Source: CAD feature listing. Evaluate the final solid. Frame: model axes, mm. Give positions to 0.01 mm unless a question says otherwise; leave off trailing zeros. Loops run counter-clockwise (first coordinate to the right, second up) from the corner with the lowest first, then second, coordinate; pieces in that order, holes last. Notation, with made-up numbers: M -31,29.5 L -12,29.5 A11 ccw -12,49.5 Z; hole C 57,73.5 d7. An arc over 180 degrees is marked long. Put each result on its own line as item: value.
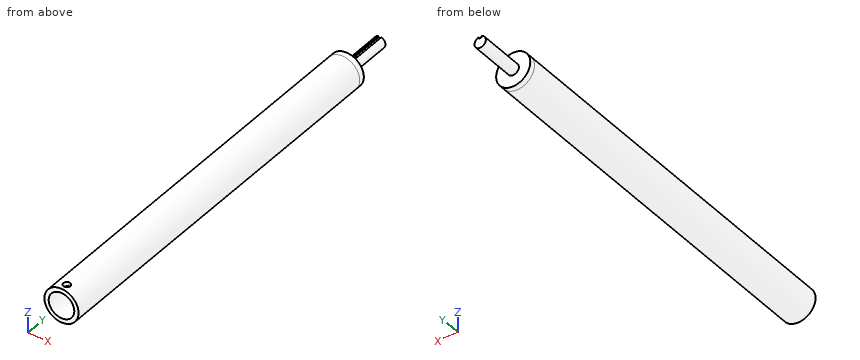
from build123d import *

# Parameters (mm, degrees)
F0_R      = 19.05
F0_R_2    = 14.2875
F1_DEPTH  = 431.8
F2_R      = 19.05
F3_DEPTH  = 6.35
F4_R      = 6.35
F5_DEPTH  = 50.8
F6_W      = 1.6129
F6_H      = 1.778
F7_DEPTH  = 38.1
F10_DEPTH = 9.525


with BuildPart() as f1:
    # F0 (on Front) → F1 (new body)
    with BuildSketch(Plane.XZ):
        Circle(F0_R)
        Circle(F0_R_2, mode=Mode.SUBTRACT)
    extrude(amount=F1_DEPTH)

    # F2 (on face) → F3 (join)
    with BuildSketch(Plane(origin=(0, 0, 0), x_dir=(-1, 0, 0), z_dir=(0, 1, 0))):
        Circle(F2_R)
    extrude(amount=F3_DEPTH)

    # F4 (on face) → F5 (join)
    with BuildSketch(Plane(origin=(0, 6.35, 0), x_dir=(-1, 0, 0), z_dir=(0, 1, 0))):
        Circle(F4_R)
    extrude(amount=F5_DEPTH)

    # F6 (on face) → F7 (cut)
    with BuildSketch(Plane(origin=(0, 57.15, 0), x_dir=(-1, 0, 0), z_dir=(0, 1, 0))):
        with Locations((-0.80645, 5.461)):
            Rectangle(F6_W, F6_H)
        with Locations((0.80645, 5.461)):
            Rectangle(F6_W, F6_H)
    extrude(amount=-F7_DEPTH, mode=Mode.SUBTRACT)

    # F9 (on offset) → F10 (cut)
    with BuildSketch(Plane.XY.offset(19.05)):
        with BuildLine():
            ThreePointArc((0, -419.89375), (-2.80633, -426.66883), (3.96875, -423.8625))
            ThreePointArc((3.96875, -423.8625), (2.80633, -421.05617), (0, -419.89375))
        make_face()
    extrude(amount=-F10_DEPTH, mode=Mode.SUBTRACT)


solid = f1.part
1. Section query A-A (z = 0). Output: boundary loops of the cut face in (x, y), plus the area to 3 significant figures.
Found:
outline: M -19.05,-431.8 L -14.29,-431.8 L -14.29,0 L 14.29,0 L 14.29,-431.8 L 19.05,-431.8 L 19.05,6.35 L 6.35,6.35 L 6.35,57.15 L -6.35,57.15 L -6.35,6.35 L -19.05,6.35 Z
area: 5,000 mm^2
2. Material intervals for line 1 (X direction, y = -232, z = 0.5); line 2 (Z direction, x = 0, y = -215); line 3 (Y direction, x = -13, z = -5), sorted ascending. Write a range as from..to.
Found:
line 1: -19.04..-14.28, 14.28..19.04
line 2: -19.05..-14.29, 14.29..19.05
line 3: 0..6.35
3. Contact query for flat-ended pins moving along their axis: P1, Ø3, axis at x = 5, z = 1.5, coming from the -Y side; P2, Ø5, axis at y = -190.5, z = -7, coming from the -X side; P3, Ø12.5, axis at x = 0, y = -423.86, coming from the -Z side; P4, Ø14.5, axis at x = 2.5, z = -7, coming from the -Y side. Output: stop coordinate, or through.
Found:
P1: y = 0
P2: x = -18.51
P3: z = -19.05
P4: y = -431.8
